Design review of the part built by this model. Coordinates are the model's own, in mm. A direction names the side the tool comes from. Give positions to 0.01 mm unless a question says otherwise; leave off trailing zeros. Loops run counter-clockwise (first coordinate to the right, second up) from the corner with the lowest first, then second, coordinate; pieces in that order, holes last.
from build123d import *

# Parameters (mm, degrees)
BOSS_EXTRUDE1_DEPTH = 50
SKETCH2_R           = 25
BOSS_EXTRUDE2_DEPTH = 10


with BuildPart() as part:
    # Sketch1 → Boss-Extrude1 (new body)
    with BuildSketch(Plane.XY):
        with BuildLine():
            Line((25, 25), (25, -25))
            Line((25, -25), (-25, -25))
            Line((-25, -25), (-25, 25))
            ThreePointArc((-25, 25), (0, 22.474363409), (25, 25))
        make_face()
    extrude(amount=BOSS_EXTRUDE1_DEPTH)

    # Sketch2 → Boss-Extrude2 (add)
    with BuildSketch(Plane.XZ.offset(25)):
        with Locations((0, 25)):
            Circle(SKETCH2_R)
    extrude(amount=BOSS_EXTRUDE2_DEPTH)


solid = part.part
Q1. Take a section at C-C (y = -29). Give the boundary of the cut face in (x, z).
Results:
outline: circle Ø50 at (0, 25)
Q2. Take a section at A-A (z = 46). Give the boundary of the cut face in (x, y), plus the area to 3 significant figures.
Results:
outline: (-25, -25) - (-13.56, -25) - (-13.56, -35) - (13.56, -35) - (13.56, -25) - (25, -25) - (25, 25) arc R124.99 cw to (-25, 25) - close
area: 2,690 mm2
Q3. Insertion check: pin 1 (3 mm diameter, centred on x = -8, z = 29, fed in from +Y); pin 2 (4 mm diameter, centred on x = -9.5, z = 30, fed in from +Y); pin 3 (8 mm diameter, centred on x = 0, z = 34, fed in from +Y). Each pin has a flat end and moves straight along its axis. Give the tip position at first contact, or say it passes through.
Results:
pin 1: stops at y = 22.84
pin 2: stops at y = 23
pin 3: stops at y = 22.54
Q4. Wall thickness on line 1 (Y direction, x = 6, z = 41.5); line 2 (Y direction, x = 7, z = 34.5): over which ranges is each line inside the solid? List them lowest first.
Results:
line 1: y = -35 to 22.62
line 2: y = -35 to 22.67
Q5. Tool access review of faces 1 (the face through (-19, -25, 5)), 2 (the face through (20, -25, 6)), 3 (the face through (20, -25, 44)), 4 (the face through (-20, -25, 45)): name each direction out of +Z, -Z, +X, -X, +Y, -Y from which nothing blocks a thin tool from reaching the whole face with its end or side.
Results:
face 1: -Z, -X, -Y
face 2: -Z, +X, -Y
face 3: +Z, +X, -Y
face 4: +Z, -X, -Y
Q6. Take a section at B-B (x = -6). Give the boundary of the cut face in (y, z), plus the area to 3 significant figures.
Results:
outline: (-35, 0.73) - (-25, 0.73) - (-25, 0) - (22.62, 0) - (22.62, 50) - (-25, 50) - (-25, 49.27) - (-35, 49.27) - close
area: 2,870 mm2
